The model under review builds one solid part; all positions refer to its coordinate system, in mm. A direction names the side the tool comes from. Give positions to 0.01 mm unless a question says otherwise; leave off trailing zeros. Order: outer loops, then holes, each group sorted by start corner. A loop starts at its lowest first (then second) coordinate and runs counter-clockwise, first axis right, second up. Notation, with made-up numbers: (50.25, 30) - (68.25, 30) arc R18 ccw to (68.25, 60) - close; hole circle Ø6 at (1.5, 36.25). An arc over 180 degrees is marked (long way). Put each result on its own line as item: value.
```python
from build123d import *

# Parameters (mm, degrees)
F0_R           = 10.9
F1_DEPTH       = 7
F2_SIZE2       = 0.4
F2_SIZE        = 0.2
F3_R           = 2
F4_R           = 4
F5_DEPTH       = 3
F7_D           = 5
F7_DEPTH       = 10
F7_CBORE_D     = 8
F7_CBORE_DEPTH = 4.2
F8_R           = 6
F8_R_2         = 2
F9_DEPTH       = 1


with BuildPart() as f1:
    # F0 (on Top) → F1 (new body)
    with BuildSketch(Plane.XY):
        Circle(F0_R)
    extrude(amount=F1_DEPTH)

    # F2
    f2_edges = [f1.edges().sort_by_distance(p)[0] for p in [
        (-10.9, 0, 0),
    ]]
    chamfer(f2_edges, length=F2_SIZE, length2=F2_SIZE2)

    # F3
    f3_edges = [f1.edges().sort_by_distance(p)[0] for p in [
        (-10.9, 0, 7),
    ]]
    fillet(f3_edges, radius=F3_R)

    # F4 (on face) → F5 (join)
    with BuildSketch(Plane(origin=(0, 0, 0), x_dir=(1, 0, 0), z_dir=(0, 0, -1))):
        Circle(F4_R)
    extrude(amount=F5_DEPTH)

    # F7
    with Locations(Plane.XY.offset(7)):
        with Locations((0, 0)):
            CounterBoreHole(F7_D / 2, F7_CBORE_D / 2, F7_CBORE_DEPTH, depth=F7_DEPTH)

    # F8 (on face) → F9 (join)
    with BuildSketch(Plane(origin=(0, 0, 0), x_dir=(1, 0, 0), z_dir=(0, 0, -1))):
        Circle(F8_R)
        Circle(F8_R_2, mode=Mode.SUBTRACT)
    extrude(amount=F9_DEPTH)


solid = f1.part
```
(1) Take a section at C-C, the plane z = -1.75. Write out the cut boundary in (x, y).
The answers:
outline: circle Ø8 at (0, 0); hole circle Ø5 at (0, 0)
(2) For faces 4 (the flat face through (-1.42, 3.92, -1)), 5 (the flat face through (2, 2, 2.8)), 6 (the flat face through (4, -2, 7)), list the 3-axis set-ups (+Z, -Z, +X, -X, +Y, -Y) from which the entire face can be reached by the end or side of a thin tool; tool diameter is ignored.
The answers:
face 4: -Z
face 5: +Z
face 6: +Z, +X, -X, +Y, -Y
(3) Wall thickness on L1, parallel to X at y = 0, z = -0.55; L2, parallel to Y at x = 0, z = 0.9; L3, parallel to Z at x = 2, y = -7.5: over which ranges is each line inside the solid? List them lowest first.
The answers:
L1: -6 to -2, 2 to 6
L2: -10.9 to -2.5, 2.5 to 10.9
L3: 0 to 7
(4) Clearance check with flat-ended pins moving along their axes: pin 1 Ø1.5 at (y, z) = (7, 5.5) entering from -X; pin 2 Ø4 at (y, z) = (-8.5, 1) entering from +X; pin 3 Ø1.5 at (y, z) = (4, 0.5) entering from -X. State where each tip first meets the part, or that it passes through.
The answers:
pin 1: x = -8.88
pin 2: x = 8.75
pin 3: x = -10.4
(5) Take a section at D-D, the plane z = 1.5. Write out the cut boundary in (x, y), then the cut area to 3 significant figures.
The answers:
outline: circle Ø21.8 at (0, 0); hole circle Ø5 at (0, 0)
area: 354 mm^2
(6) The part is to be moulded in two halves that separate along Y. For faces 1 (the cylindrical face through (-5.994, -0.264, -0.493)), 2 (the cylindrical face through (-0.434, 1.952, -0.493)), 3 (the flat face through (2, -2, -3)), say which applies: pulls with the +Y half, pulls with the -Y half, needs draft (parallel to the pull), parting line crosses it, or undercut.
The answers:
face 1: parting line crosses it
face 2: undercut
face 3: needs draft
